The listing builds one solid part. Answer for the finished solid, in the listing's coordinates (mm). A direction names the side the tool comes from. Coordinates: 2 decimals unless noted, no trailing zeros. Loops run counter-clockwise (first coordinate to the right, second up) from the corner with the lowest first, then second, coordinate; pieces in that order, holes last. Notation, with made-up numbers: (-1.75, -30.5) - (44.25, -30.5) arc R18 cw to (44.25, -25.5) - close; hole circle Ø11 at (48.5, 37). An arc over 180 degrees is marked (long way). Return JSON: item names as keys, results as strings. Group by question number.
1. Each of these flat-tipped pins is pushed along its axis until it touches: P1, Ø10, axis at x = 61, y = 7.5, coming from the -Z side; P2, Ø1.9, axis at x = 76, y = 19.5, coming from the +Z side. Where does it stop, or does it pass through?
2. Section B-B (y = 21.5) is taken. Write down the section's boundary in (x, z), and give its area (3 significant figures).
3. Section D-D (y = 16) is taken. Write down the section's boundary in (x, z).
4. Find the intervals of material crossed by line 1 along X through (y, z) = (18.5, 10.5); line 2 along Z through (x, y) = (72.5, 21.5); line 3 along Y through (x, z) = (23, 13.5), in increasing order.
5. Section C-C (y = 3.5) is taken. Write down the section's boundary in (x, z).
6. The mould has two halves that part along X. Classify faces 3 (the face through (75.68, 18.78, 1.48)), 4 (the face through (71.41, 36.36, 6.68)), 5 (the face through (36.47, 0.57, 14.58)), 6 (the face through (-6.185, 18.558, 1.479)): pulls with the +X half, pulls with the -X half, needs draft (parallel to the pull), parting line crosses it, or undercut.
7. Which of the six approach directions +Z, -Z, +X, -X, +Y, -Y give full straight-line access (tool end or side, diameter ignored) to faces 1 (the face through (73.709, 13.074, 1.479)), 2 (the face through (74, 17, 3))?
8. Section A-A (z = 11.75) is taken. Write down the section's boundary in (x, y).
```python
from build123d import *

# Parameters (mm, degrees)
F1_DEPTH = 15.18412
F0_R     = 1
F2_DEPTH = 3
F3_R     = 2


with BuildPart() as f1:
    # F0 (on Top) → F1 (new body)
    with BuildSketch(Plane.XY):
        Polygon((0, 12.4455), (0, 0), (71.9836, 0), (71.9836, 12.4455), (71.9836, 24.511), (71.9836, 36.957), (0, 36.957), (0, 24.511), align=None)
    extrude(amount=F1_DEPTH)

    # F0 (on Top) → F2 (join)
    with BuildSketch(Plane.XY):
        with BuildLine():
            Line((71.9836, 24.511), (71.9836, 12.4455))
            Line((71.9836, 12.4455), (75.4836, 13.719396))
            ThreePointArc((75.4836, 13.719396), (78.1688, 18.47825), (75.4836, 23.237104))
            Line((75.4836, 23.237104), (71.9836, 24.511))
        make_face()
        with Locations((74.7268, 18.4785)):
            Circle(F0_R, mode=Mode.SUBTRACT)
        with BuildLine():
            Line((-3.5, 13.719396), (0, 12.4455))
            Line((0, 12.4455), (0, 24.511))
            Line((0, 24.511), (-3.5, 23.237104))
            ThreePointArc((-3.5, 23.237104), (-6.1852, 18.47825), (-3.5, 13.719396))
        make_face()
        with Locations((-2.7432, 18.4785)):
            Circle(F0_R, mode=Mode.SUBTRACT)
    extrude(amount=F2_DEPTH)

    # F3
    f3_edges = [f1.edges().sort_by_distance(p)[0] for p in [
        (0, 18.4785, 15.18412),
        (35.9918, 0, 15.18412),
        (71.9836, 18.4785, 15.18412),
        (35.9918, 36.957, 15.18412),
        (0, 36.957, 7.59206),
        (71.9836, 36.957, 7.59206),
        (71.9836, 0, 7.59206),
        (0, 0, 7.59206),
    ]]
    fillet(f3_edges, radius=F3_R)


solid = f1.part
```
The answers:
{
 "1": {"P1": "stops at z = 0", "P2": "stops at z = 3"},
 "2": {"outline": "(-5.29, 0) - (77.28, 0) - (77.28, 3) - (71.98, 3) - (71.98, 13.18) arc R2 ccw to (69.98, 15.18) - (2, 15.18) arc R2 ccw to (0, 13.18) - (0, 3) - (-5.29, 3) - close", "area": "1,120 mm2"},
 "3": {"outline": "(-5.6, 0) - (77.59, 0) - (77.59, 3) - (71.98, 3) - (71.98, 13.18) arc R2 ccw to (69.98, 15.18) - (2, 15.18) arc R2 ccw to (0, 13.18) - (0, 3) - (-5.6, 3) - close"},
 "4": {"line 1": "x = 0 to 71.98", "line 2": "z = 0 to 3", "line 3": "y = 0.03 to 36.93"},
 "5": {"outline": "(0, 0) - (71.98, 0) - (71.98, 13.18) arc R2 ccw to (69.98, 15.18) - (2, 15.18) arc R2 ccw to (0, 13.18) - close"},
 "6": {"face 3": "undercut", "face 4": "pulls with the +X half", "face 5": "needs draft", "face 6": "pulls with the -X half"},
 "7": {"face 1": "+Z, -Z, +X, -Y", "face 2": "+Z, +X, +Y, -Y"},
 "8": {"outline": "(0, 2) arc R2 ccw to (2, 0) - (69.98, 0) arc R2 ccw to (71.98, 2) - (71.98, 34.96) arc R2 ccw to (69.98, 36.96) - (2, 36.96) arc R2 ccw to (0, 34.96) - close"}
}
